from build123d import *

# Parameters (mm, degrees)
F0_W     = 110
F0_H     = 60
F0_W_2   = 65
F0_H_2   = 30
F1_DEPTH = 19
F2_W     = 110
F2_H     = 42
F2_W_2   = 65
F2_H_2   = 30
F3_DEPTH = 12
F4_W     = 15
F4_H     = 15
F5_DEPTH = 2
F6_R     = 3
F8_D     = 5.5
F8_DEPTH = 50
F9_D     = 8.4
F9_DEPTH = 50


with BuildPart() as f1:
    # F0 (on Front) → F1 (new body)
    with BuildSketch(Plane.XZ):
        with Locations((55, 30)):
            Rectangle(F0_W, F0_H)
        with Locations((49.5, 30)):
            Rectangle(F0_W_2, F0_H_2, mode=Mode.SUBTRACT)
    extrude(amount=F1_DEPTH)

    # F2 (on face) → F3 (cut)
    with BuildSketch(Plane(origin=(0, 0, 0), x_dir=(-1, 0, 0), z_dir=(0, 1, 0))):
        with Locations((-55, 30)):
            Rectangle(F2_W, F2_H)
        with Locations((-49.5, 30)):
            Rectangle(F2_W_2, F2_H_2, mode=Mode.SUBTRACT)
    extrude(amount=-F3_DEPTH, mode=Mode.SUBTRACT)

    # F4 (on face) → F5 (cut)
    with BuildSketch(Plane.XZ.offset(19)):
        Polygon((20, 60), (0, 60), (0, 0), (20, 0), (20, 15), (17, 15), (17, 45), (20, 45), align=None)
        with Locations((97, 30)):
            Rectangle(F4_W, F4_H)
    extrude(amount=-F5_DEPTH, mode=Mode.SUBTRACT)

    # F6
    f6_edges = [f1.edges().sort_by_distance(p)[0] for p in [
        (17, -14.5, 45),
        (17, -14.5, 15),
        (82, -15.5, 45),
        (82, -15.5, 15),
        (89.5, -18, 37.5),
        (104.5, -18, 37.5),
        (104.5, -18, 22.5),
        (89.5, -18, 22.5),
    ]]
    fillet(f6_edges, radius=F6_R)

    # F8
    with Locations(Plane.XZ.offset(17)):
        with Locations((10, 45), (10, 15)):
            Hole(F8_D / 2, depth=F8_DEPTH)

    # F9
    with Locations(Plane.XZ.offset(17)):
        with Locations((97, 30)):
            Hole(F9_D / 2, depth=F9_DEPTH)


solid = f1.part
The model under review builds one solid part; all positions refer to its coordinate system, in mm. A direction names the side the tool comes from. Round coordinates to 2 decimals unless told otherwise and drop trailing zeros. Write each loop counter-clockwise with the first axis right and the second up, starting at its lowest first coordinate (ties: lowest second). Pieces come first, ordered by that corner, then holes. Notation, with made-up numbers: M 53,87 L 97,87 A15 cw 97,114 Z; hole C -26,80 d10. An arc over 180 degrees is marked long. Use a Markdown table: item, result. Add a question column.
Q1. We need section A-A, the plane z = 30. State the section outline as (x, y) points.
Q2. Machinability: for faces 4 (the face through (10, -17, 30)), 5 (the face through (17.86, -14.54, 44.1)), 6 (the face through (90.4, -17.99, 36.64)), which of the approach directions +Z, -Z, +X, -X, +Y, -Y give a long, thin tool a straight path to every point of the face, cutting with its end or side? Answer none if there is none.
Q3. To check wall thickness, follow line 1 (Z direction, x = 10, y = -15.4); line 2 (Z direction, x = 52, y = -7.5); line 3 (Z direction, x = 97, y = -14). State the ranges of each line that lie inside material, in increasing order.
Q4. The part is to be moulded in two halves that separate along Z. For faces 1 (the face through (54, -9, 60)), 2 (the face through (54, -9, 0)), 3 (the face through (81.1, -15.55, 15.86)), say which applies: pulls with the +Z half, pulls with the -Z half, needs draft (parallel to the pull), parting line crosses it, or undercut.
Q5. We need section B-B, the plane x = 53. State the section outline as (y, z) points, plus the area to 3 significant figures.
Q6. We need section C-C, the plane y = -8. State the section outline as (x, z) points, plus the area to 3 significant figures.
Q7. Insertion check: pin 1 (9 mm diameter, centred on x = 10, z = 45, fed in from -Y); pin 2 (1.6 mm diameter, centred on y = -18.5, z = 52.5, fed in from -X); pin 3 (6.5 mm diameter, centred on x = 97, z = 30, fed in from -Y). Each pin has a flat end and moves straight along its axis. Give the tip position at first contact, or say it passes through.
Q8. We need section D-D, the plane x = 10. State the section outline as (y, z) points, plus the area to 3 significant figures.
Findings below:
| question | item | result |
|---|---|---|
| 1 | outline | M 0,-17 L 17,-17 L 17,-12 L 0,-12 Z; M 82,-19 L 89.5,-19 L 89.5,-17 L 92.8,-17 L 92.8,-12 L 82,-12 Z; M 101.2,-17 L 104.5,-17 L 104.5,-19 L 110,-19 L 110,-12 L 101.2,-12 Z |
| 2 | face 4 | +Z, -Z, -X, -Y |
| 2 | face 5 | +Y, -Y |
| 2 | face 6 | -Y |
| 3 | line 1 | z = 0 to 12.25, 17.75 to 42.25, 47.75 to 60 |
| 3 | line 2 | z = 0 to 9, 51 to 60 |
| 3 | line 3 | z = 0 to 25.8, 34.2 to 60 |
| 4 | face 1 | pulls with the +Z half |
| 4 | face 2 | pulls with the -Z half |
| 4 | face 3 | undercut |
| 5 | outline | M -19,0 L 0,0 L 0,9 L -12,9 L -12,15 L -19,15 Z; M -19,45 L -12,45 L -12,51 L 0,51 L 0,60 L -19,60 Z |
| 5 | area | 426 mm² |
| 6 | outline | M 0,0 L 110,0 L 110,9 L 0,9 Z; M 0,51 L 110,51 L 110,60 L 0,60 Z |
| 6 | area | 1,980 mm² |
| 7 | pin 1 | stops at y = -17 |
| 7 | pin 2 | stops at x = 20 |
| 7 | pin 3 | passes through |
| 8 | outline | M -17,0 L 0,0 L 0,9 L -12,9 L -12,12.25 L -17,12.25 Z; M -17,17.75 L -12,17.75 L -12,42.25 L -17,42.25 Z; M -17,47.75 L -12,47.75 L -12,51 L 0,51 L 0,60 L -17,60 Z |
| 8 | area | 461 mm² |
